The drawing under review shows one solid part. Ordinate dimensions are in mm from its lowest x, y, z. Give positions to 0.01 mm unless a question says otherwise; leave off trailing zeros. Order: outer loops, then holes, each group sorted by start corner. A loop starts at its lowest first (then second) coordinate and runs counter-clockwise, first axis right, second up. Notation, with made-up numbers: (46, 29) - (66, 29) arc R24 ccw to (66, 62) - close; hole circle Ø5 at (56, 34.25). An arc over 180 degrees is marked (long way). Write item = value, one per line. Start each with the question number.
1. We need section A-A, the plane z = 0.95. Give the boundary of the cut face in (x, y).
2. We need section B-B, the plane y = 7.25. Give the boundary of the cut face in (x, z).
3. Wall thickness on probe 1 along Z at (x, y) = (6.25, 7); probe 2 along Y at (x, z) = (0.5, 1); probe 3 along X at (y, z) = (3.75, 0.9): over which ranges is each line inside the solid? List them lowest first.
4. We need section D-D, the plane x = 5. Give the boundary of the cut face in (y, z), and give its area (3 significant figures).
5. We need section C-C, the plane x = 9.25. Give the boundary of the cut face in (y, z).
6. Mouldability with a two-part tool opening along X and no side actions: class the marked faces 1 and 2 as pulls with the +X half, pulls with the -X half, needs draft (parallel to the pull), parting line crosses it, or undercut.
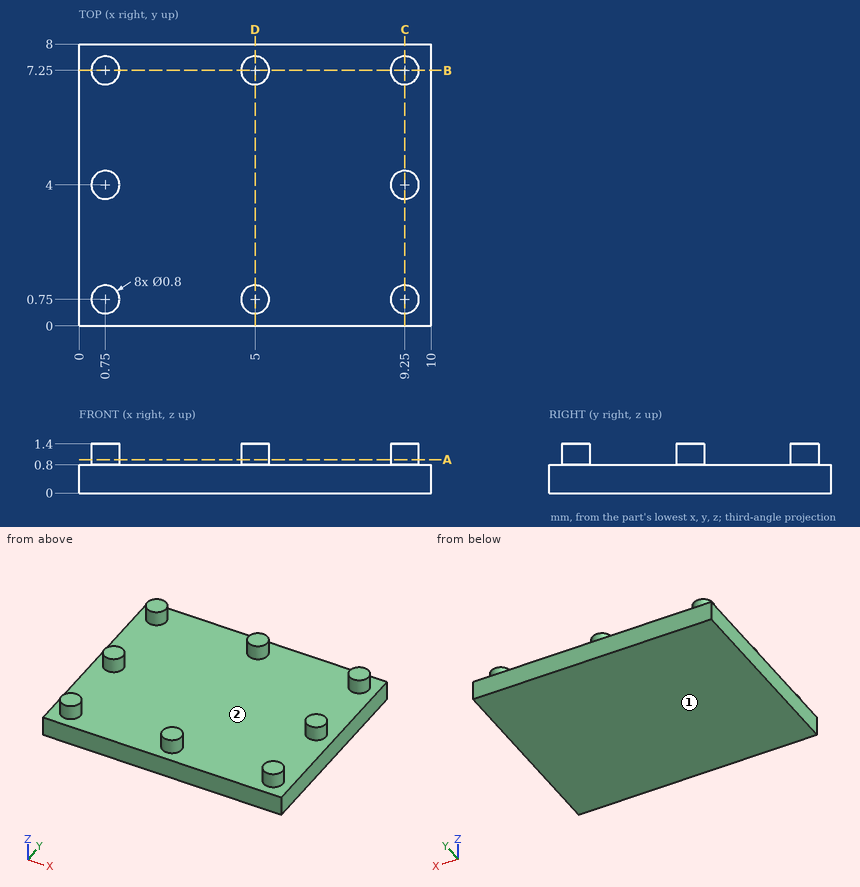
Model answer:
q1.outline = circle Ø0.8 at (0.75, 0.75); circle Ø0.8 at (0.75, 4); circle Ø0.8 at (0.75, 7.25); circle Ø0.8 at (5, 0.75); circle Ø0.8 at (5, 7.25); circle Ø0.8 at (9.25, 0.75); circle Ø0.8 at (9.25, 4); circle Ø0.8 at (9.25, 7.25)
q2.outline = (0, 0) - (10, 0) - (10, 0.8) - (9.65, 0.8) - (9.65, 1.4) - (8.85, 1.4) - (8.85, 0.8) - (5.4, 0.8) - (5.4, 1.4) - (4.6, 1.4) - (4.6, 0.8) - (1.15, 0.8) - (1.15, 1.4) - (0.35, 1.4) - (0.35, 0.8) - (0, 0.8) - close
q3.probe_1 = 0 to 0.8
q3.probe_2 = 0.44 to 1.06, 3.69 to 4.31, 6.94 to 7.56
q3.probe_3 = 0.44 to 1.06, 8.94 to 9.56
q4.outline = (0, 0) - (8, 0) - (8, 0.8) - (7.65, 0.8) - (7.65, 1.4) - (6.85, 1.4) - (6.85, 0.8) - (1.15, 0.8) - (1.15, 1.4) - (0.35, 1.4) - (0.35, 0.8) - (0, 0.8) - close
q4.area = 7.36 mm2
q5.outline = (0, 0) - (8, 0) - (8, 0.8) - (7.65, 0.8) - (7.65, 1.4) - (6.85, 1.4) - (6.85, 0.8) - (4.4, 0.8) - (4.4, 1.4) - (3.6, 1.4) - (3.6, 0.8) - (1.15, 0.8) - (1.15, 1.4) - (0.35, 1.4) - (0.35, 0.8) - (0, 0.8) - close
q6.face_1 = needs draft
q6.face_2 = undercut
